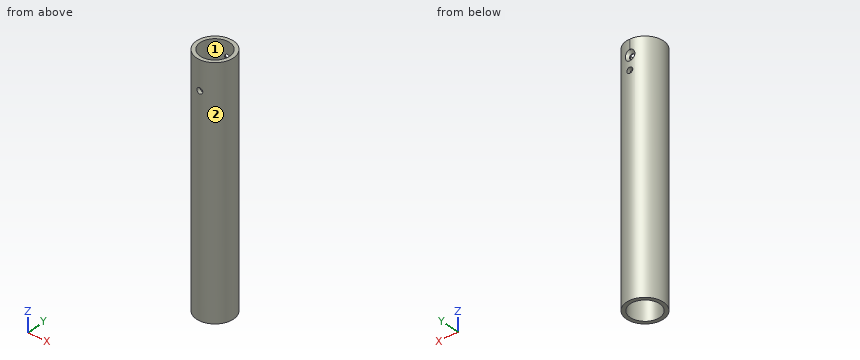
from build123d import *

# Parameters (mm, degrees)
SKETCH1_R                     = 12.5
SKETCH1_R_2                   = 10
BOSS_EXTRUDE1_DEPTH           = 163.5
CSK_FOR_M3_SFHCS1_D           = 3.4
CSK_FOR_M3_SFHCS1_DEPTH       = 10
CSK_FOR_M3_SFHCS1_CSINK_D     = 7.22
CSK_FOR_M3_SFHCS1_CSINK_ANGLE = 90
CSK_FOR_M3_SFHCS1_TIP         = 1.021463052
F_4_0MM_DOWEL_HOLE1_D         = 4
SKETCH8_W                     = 10
SKETCH8_H                     = 0.5
CUT_EXTRUDE1_DEPTH            = 0.25


with BuildPart() as part:
    # Sketch1 → Boss-Extrude1 (new body)
    with BuildSketch(Plane.XY):
        Circle(SKETCH1_R)
        Circle(SKETCH1_R_2, mode=Mode.SUBTRACT)
    extrude(amount=-BOSS_EXTRUDE1_DEPTH)

    # CSK for M3 SFHCS1
    with Locations(Plane.ZX.offset(12.5)):
        with Locations((-10, 0)):
            CounterSinkHole(CSK_FOR_M3_SFHCS1_D / 2, CSK_FOR_M3_SFHCS1_CSINK_D / 2, depth=CSK_FOR_M3_SFHCS1_DEPTH, counter_sink_angle=CSK_FOR_M3_SFHCS1_CSINK_ANGLE)
            with Locations((0, 0, -(CSK_FOR_M3_SFHCS1_DEPTH + CSK_FOR_M3_SFHCS1_TIP / 2))):  # 118° drill point
                Cone(0, CSK_FOR_M3_SFHCS1_D / 2, CSK_FOR_M3_SFHCS1_TIP, mode=Mode.SUBTRACT)

    # Ø4.0mm Dowel Hole1 (through all)
    with Locations(Plane.ZX.offset(12.5)):
        with Locations((-19.5, 0)):
            Hole(F_4_0MM_DOWEL_HOLE1_D / 2)

    # Sketch8 → Cut-Extrude1 (cut)
    with BuildSketch(Plane.ZX.offset(12.5)):
        with Locations((-5, 0)):
            Rectangle(SKETCH8_W, SKETCH8_H)
    extrude(amount=-CUT_EXTRUDE1_DEPTH, mode=Mode.SUBTRACT)


solid = part.part
Input: part model. Units: mm. Frame: model coordinates. Face numbers are marked on the shaded views. Coordinates: 2 decimals unless noted, no trailing zeros. Write each loop counter-clockwise with the first axis right and the second up, starting at its lowest first coordinate (ties: lowest second). Pieces come first, ordered by that corner, then holes. Notation, with made-up numbers: M -30,-11.5 L -22,-11.5 A29 ccw -22,14.5 Z; hole C 59,22.25 d3. An arc over 180 degrees is marked long. Answer as a JSON object with one key per item and string values. Group by question number.
(1) Contact query for flat-ended pins moving along their axis: P1, Ø3, axis at x = 1, y = -6.5, coming from the -Z side; P2, Ø8, axis at y = 8.5, z = -24.5, coming from the -X side; P3, Ø1, axis at x = 4.5, z = -141.5, coming from the -Y side; P4, Ø1, axis at y = 8.5, z = -121.5, coming from the +X side. Output: stop coordinate, or through.
(2) Section D-D on z = -10. Output: boundary loops of the cut face in (x, y).
(3) Ray query, line 1 along X through (y, z) = (0.25, -59); line 2 along Z through (x, y) = (0, -11.35); line 3 along Y through (x, z) = (0.75, -128). Return the intervals inside material, ascending. Write a range as [from, to].
(4) Section B-B on x = -7.25. Output: boundary loops of the cut face in (y, z), plus the area to 3 significant figures.
(5) Mould query, pull axis Y, two halves, no side actions, for the marked faces 1 and 2. Classes: pulls with the +Y half, pulls with the -Y half, needs draft (parallel to the pull), parting line crosses it, or undercut.
(6) Section C-C on z = -51. Output: boundary loops of the cut face in (x, y), plus the area to 3 significant figures.
(7) Section A-A on y = 0. Output: boundary loops of the cut face in (x, z), plus the area to 4 significant figures.
Result set:
{
 "1": {"P1": "passes through", "P2": "stops at x = -11.66", "P3": "stops at y = -11.84", "P4": "stops at x = 9.6"},
 "2": {"outline": "M -3.19,12.08 A12.5 ccw long 3.19,12.08 L 1.7,10.59 L 1.7,9.85 A10 cw long -1.7,9.85 L -1.7,10.59 Z"},
 "3": {"line 1": "x = [-12.5, -10], [10, 12.5]", "line 2": "z = [-163.5, -21.5], [-17.5, 0]", "line 3": "y = [-12.48, -9.97], [9.97, 12.48]"},
 "4": {"outline": "M -10.18,-163.5 L -6.89,-163.5 L -6.89,0 L -10.18,0 Z; M 6.89,-163.5 L 10.18,-163.5 L 10.18,0 L 6.89,0 Z", "area": "1,080 mm2"},
 "5": {"face 1": "undercut", "face 2": "parting line crosses it"},
 "6": {"outline": "C 0,0 d25; hole C 0,0 d20", "area": "177 mm2"},
 "7": {"outline": "M -12.5,-163.5 L -10,-163.5 L -10,0 L -12.5,0 Z; M 10,-163.5 L 12.5,-163.5 L 12.5,0 L 10,0 Z", "area": "817.5 mm2"}
}
